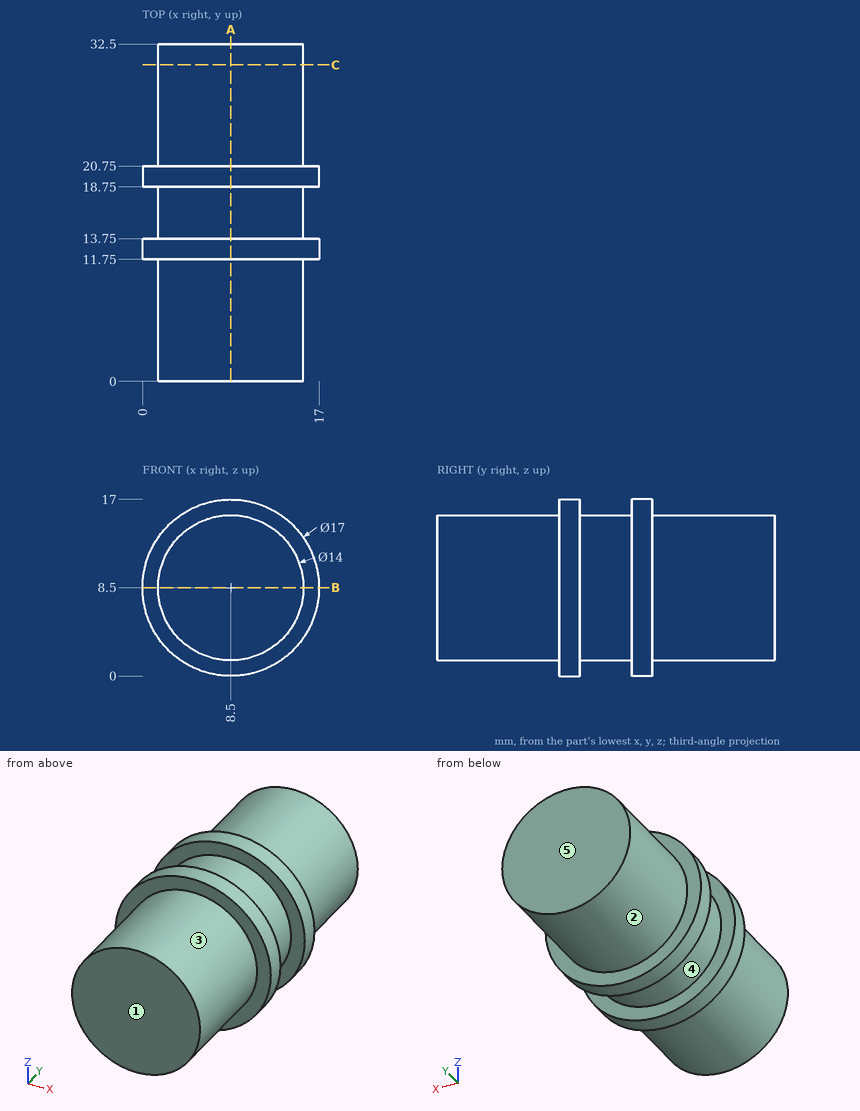
Design review of the part shown in the three views and the two pictorial views. Dimensions are in mm from the part's minimum x, y and z. A direction names the side the tool comes from. Coordinates: 2 decimals unless noted, no trailing zeros. Loops run counter-clockwise (first coordinate to the right, second up) from the corner with the lowest first, then second, coordinate; pieces in that order, holes last. Notation, with made-up numbers: M 17.5,84.25 L 44.5,84.25 A28 ccw 44.5,104.25 Z; hole C 5,77.25 d1. An arc over 180 degrees is marked long. One line per question, with ' | ' between items.
(1) Wall thickness on probe 1 along Y at (x, z) = (14.5, 12.75); probe 2 along Z at (x, y) = (8.5, 9.5); probe 3 along X at (y, z) = (12, 8.75): over which ranges is each line inside the solid? List them lowest first.
Filled in:
probe 1: y = 11.75 to 13.75, 18.75 to 20.75 | probe 2: z = 1.5 to 15.5 | probe 3: x = 0 to 17
(2) Draft analysis for pull direction Y (two halves, no side actions). For the marked faces 3, 4 and 5, state which applies: released by +Y, released by -Y, zero draft, split by the parting line, or undercut.
Filled in:
face 3: zero draft | face 4: undercut | face 5: released by +Y
(3) For pin 1 Ø3 at (y, z) = (4, 7.5) entering from +X; pin 2 Ø5 at (x, y) = (2, 7.5) entering from +Z; pin 3 Ø5 at (y, z) = (23, 7) entering from +X, all flat-tipped, find the tip position at first contact; note any pin that passes through.
Filled in:
pin 1: stops at x = 15.5 | pin 2: stops at z = 14.24 | pin 3: stops at x = 16.99
(4) We need section C-C (y = 30.5). Give the boundary of the cut face in (x, z), and give its area (3 significant figures).
Filled in:
outline: C 8.5,8.5 d14 | area: 154 mm^2
(5) We need section B-B (z = 8.5). Give the boundary of the cut face in (x, y).
Filled in:
outline: M 0,11.75 L 1.5,11.75 L 1.5,0 L 15.5,0 L 15.5,11.75 L 17,11.75 L 17,13.75 L 15.5,13.75 L 15.5,18.75 L 17,18.75 L 17,20.75 L 15.5,20.75 L 15.5,32.5 L 1.5,32.5 L 1.5,20.75 L 0,20.75 L 0,18.75 L 1.5,18.75 L 1.5,13.75 L 0,13.75 Z
(6) Machinability: for the marked faces 1 and 2, which of the approach directions +Z, -Z, +X, -X, +Y, -Y give a long, thin tool a straight path to every point of the face, cutting with its end or side? Answer none if there is none.
Filled in:
face 1: +Z, -Z, +X, -X, -Y | face 2: +Y
(7) We need section A-A (x = 8.5). Give the boundary of the cut face in (y, z), and give its area (3 significant figures).
Filled in:
outline: M 0,1.5 L 11.75,1.5 L 11.75,0 L 13.75,0 L 13.75,1.5 L 18.75,1.5 L 18.75,0 L 20.75,0 L 20.75,1.5 L 32.5,1.5 L 32.5,15.5 L 20.75,15.5 L 20.75,17 L 18.75,17 L 18.75,15.5 L 13.75,15.5 L 13.75,17 L 11.75,17 L 11.75,15.5 L 0,15.5 Z | area: 467 mm^2
